from build123d import *

# Parameters (mm, degrees)
ESQUISSE1_R             = 2
BOSS_EXTRU_1_DEPTH      = 13
ESQUISSE2_R             = 2.75
BOSS_EXTRU_2_DEPTH      = 1
ESQUISSE3_R             = 1.25
ENL_V_MAT_EXTRU_1_DEPTH = 14.569266745
CHANFREIN1_SIZE         = 1
CHANFREIN1_SIZE_2       = 0.577350269
CONG_2_R                = 0.5
ENL_V_MAT_EXTRU_2_DEPTH = 5


with BuildPart() as part:
    # Esquisse1 → Boss.-Extru.1 (new body)
    with BuildSketch(Plane(origin=(0, 0, 0), x_dir=(1, 0, 0), z_dir=(0, 1, 0))):
        with Locations(Location((0, 0, 0), (0, 0, 90))):
            Circle(ESQUISSE1_R)
    extrude(amount=BOSS_EXTRU_1_DEPTH)

    # Esquisse2 → Boss.-Extru.2 (add)
    with BuildSketch(Plane(origin=(0, 13, 0), x_dir=(1, 0, 0), z_dir=(0, 1, 0))):
        with Locations(Location((0, 0, 0), (0, 0, 270))):
            Circle(ESQUISSE2_R)
    extrude(amount=-BOSS_EXTRU_2_DEPTH)

    # Esquisse3 → Enlèv. mat.-Extru.1 (cut, through all)
    with BuildSketch(Plane(origin=(0, 13, 0), x_dir=(1, 0, 0), z_dir=(0, 1, 0))):
        with Locations(Location((0, 0, 0), (0, 0, 270))):
            Circle(ESQUISSE3_R)
    extrude(amount=-ENL_V_MAT_EXTRU_1_DEPTH, mode=Mode.SUBTRACT)

    # Chanfrein1
    # the kernel refuses this chamfer: 1, 0.577350269 mm, written as the material it takes off along each edge
    with BuildSketch(Plane(origin=(0, 13, 0), x_dir=(0, 0, 1), z_dir=(-1, 0, 0))) as chanfrein1_piece_1:
        Polygon((2.75, -CHANFREIN1_SIZE), (2.75 - CHANFREIN1_SIZE_2, 0), (2.75, 0), align=None)
    revolve(axis=Axis((0, 13, 0), (0, 1, 0)), mode=Mode.SUBTRACT)

    # Congé2
    cong_2_edges = [part.edges().sort_by_distance(p)[0] for p in [
        (0, 0, 2),
    ]]
    fillet(cong_2_edges, radius=CONG_2_R)

    # Esquisse4 → Enlèv. mat.-Extru.2 (cut)
    with BuildSketch(Plane.XZ):
        with BuildLine():
            Line((0.25, 1.984313483), (0.25, 1.224744871))
            ThreePointArc((0.25, 1.224744871), (0, 1.25), (-0.25, 1.224744871))
            Line((-0.25, 1.224744871), (-0.25, 1.984313483))
            ThreePointArc((-0.25, 1.984313483), (0, 2), (0.25, 1.984313483))
        make_face()
        with BuildLine():
            Line((1.984313483, 0.25), (1.224744871, 0.25))
            ThreePointArc((1.224744871, 0.25), (1.25, 0), (1.224744871, -0.25))
            Line((1.224744871, -0.25), (1.984313483, -0.25))
            ThreePointArc((1.984313483, -0.25), (2, 0), (1.984313483, 0.25))
        make_face()
        with BuildLine():
            Line((-1.224744871, -0.25), (-1.984313483, -0.25))
            ThreePointArc((-1.984313483, -0.25), (-2, 0), (-1.984313483, 0.25))
            Line((-1.984313483, 0.25), (-1.224744871, 0.25))
            ThreePointArc((-1.224744871, 0.25), (-1.25, 0), (-1.224744871, -0.25))
        make_face()
        with BuildLine():
            Line((0.25, -1.224744871), (0.25, -1.984313483))
            ThreePointArc((0.25, -1.984313483), (0, -2), (-0.25, -1.984313483))
            Line((-0.25, -1.984313483), (-0.25, -1.224744871))
            ThreePointArc((-0.25, -1.224744871), (0, -1.25), (0.25, -1.224744871))
        make_face()
    extrude(amount=-ENL_V_MAT_EXTRU_2_DEPTH, mode=Mode.SUBTRACT)


solid = part.part
Input: part model. Units: mm. Frame: model coordinates. Coordinates: 2 decimals unless noted, no trailing zeros. Loops run counter-clockwise (first coordinate to the right, second up) from the corner with the lowest first, then second, coordinate; pieces in that order, holes last.
Q1. Material intervals for line 1 (Z direction, x = 0, y = 6.75); line 2 (Y direction, x = -1.6, z = 0), sorted ascending.
Q2. Contact query for flat-ended pins moving along their axis: pin 1 (0.6 mm diameter, centred on y = 2.5, z = -2, fed in from +X); pin 2 (0.8 mm diameter, centred on x = 2, y = 2.5, fed in from -Z); pin 3 (3 mm diameter, centred on x = 0, y = 9, fed in from -Z). Output: stop coordinate, or through.
Q3. Cut plane C-C (y = 7.75). Output: boundary loops of the cut face in (x, z), then the cut area to 3 significant figures.
Q4. Draft query along X for faces 1 (the face through (-2, 12, 1)), 2 (the face through (-0.479, 6.591, 1.155)), 3 (the face through (0.766, 6.17, -1.847)). Return one class per face: +X half, -X half, draft (parallel to the pull), parting line (faces both ways), or undercut.
Q5. Cut plane A-A (z = 0). Output: boundary loops of the cut face in (x, y), then the cut area to 3 significant figures.
Q6. Cut plane B-B (x = 0). Output: boundary loops of the cut face in (y, z).
Working result:
1. line 1: z = -2 to -1.25, 1.25 to 2
1. line 2: y = 5 to 13
2. pin 1: stops at x = 1.05
2. pin 2: stops at z = -1.2
2. pin 3: stops at z = -2
3. outline: circle Ø4 at (0, 0); hole circle Ø2.5 at (0, 0)
3. area: 7.66 mm2
4. face 1: draft
4. face 2: undercut
4. face 3: parting line
5. outline: (-2.75, 12) - (-2, 12) - (-2, 5) - (-1.25, 5) - (-1.25, 13) - (-2.17, 13) - close; (1.25, 5) - (2, 5) - (2, 12) - (2.75, 12) - (2.17, 13) - (1.25, 13) - close
5. area: 12.9 mm2
6. outline: (5, -2) - (12, -2) - (12, -2.75) - (13, -2.17) - (13, -1.25) - (5, -1.25) - close; (5, 1.25) - (13, 1.25) - (13, 2.17) - (12, 2.75) - (12, 2) - (5, 2) - close
